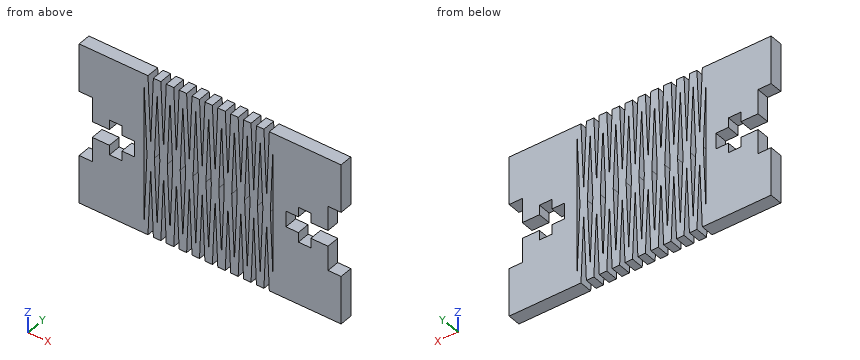
```python
from build123d import *

# Parameters (mm, degrees)
SKETCH1_W            = 61
SKETCH1_H            = 37.5
BOSS_EXTRUDE1_DEPTH  = 3
CUT_EXTRUDE2_DEPTH   = 36.927879147
MIRROR2_COPY_1_DEPTH = 36.927879147
CUT_EXTRUDE3_DEPTH   = 36.927879147
LPATTERN1_COUNT      = 10
LPATTERN1_PITCH      = 3


with BuildPart() as part:
    # Sketch1 → Boss-Extrude1 (new body)
    with BuildSketch(Plane(origin=(0, 0, 0), x_dir=(1, 0, 0), z_dir=(0, 1, 0))):
        Rectangle(SKETCH1_W, SKETCH1_H)
    extrude(amount=BOSS_EXTRUDE1_DEPTH)

    # Sketch3 → Cut-Extrude2 (cut, through all)
    with BuildSketch(Plane(origin=(0, 3, 0), x_dir=(1, 0, 0), z_dir=(0, 1, 0))):
        Polygon((30.5, 7.55), (27.45, 7.55), (27.45, 1.85), (23.45, 1.85), (23.45, 4.1), (20.55, 4.1), (20.55, 1.85), (17.65, 1.85), (17.65, 0), (30.5, 0), align=None)
    cut_extrude2 = extrude(amount=-CUT_EXTRUDE2_DEPTH, mode=Mode.SUBTRACT)

    # Mirror1: Cut-Extrude2 across plane
    add(cut_extrude2.mirror(Plane.XY), mode=Mode.SUBTRACT)

    # Mirror2: Cut-Extrude2 across plane
    add(cut_extrude2.mirror(Plane(origin=(0, 0, 0), x_dir=(0, 0, 1), z_dir=(1, 0, 0))), mode=Mode.SUBTRACT)

    # Mirror2 copy 1 sketch → Mirror2 copy 1 (cut, through all)
    with BuildSketch(Plane(origin=(0, 3, 0), x_dir=(-1, 0, 0), z_dir=(0, 1, 0))):
        Polygon((30.5, 7.55), (27.45, 7.55), (27.45, 1.85), (23.45, 1.85), (23.45, 4.1), (20.55, 4.1), (20.55, 1.85), (17.65, 1.85), (17.65, 0), (30.5, 0), align=None)
    extrude(amount=-MIRROR2_COPY_1_DEPTH, mode=Mode.SUBTRACT)

    # Sketch4 → Cut-Extrude3 (cut, through all)
    with BuildSketch(Plane(origin=(0, 3, 0), x_dir=(1, 0, 0), z_dir=(0, 1, 0))):
        Polygon((14.65, 15.575), (14.65, -15.575), (14.0229932, 0), align=None)
        Polygon((13.7770068, 18.75), (13.15, 3.175), (12.5229932, 18.75), align=None)
        Polygon((13.15, -3.175), (12.5229932, -18.75), (13.7770068, -18.75), align=None)
        Polygon((11.65, 15.575), (11.65, -15.575), (12.2770068, 0), align=None)
    cut_extrude3 = extrude(amount=-CUT_EXTRUDE3_DEPTH, mode=Mode.SUBTRACT)

    # LPattern1: Cut-Extrude3 ×10
    with Locations(*[(-i * LPATTERN1_PITCH, 0, 0) for i in range(1, LPATTERN1_COUNT)]):
        add(cut_extrude3, mode=Mode.SUBTRACT)


solid = part.part
```
Could you check a few things on this model? Use its own coordinates, in mm. Coordinates: 2 decimals unless noted, no trailing zeros. Loops run counter-clockwise (first coordinate to the right, second up) from the corner with the lowest first, then second, coordinate; pieces in that order, holes last. Notation, with made-up numbers: M -37,6 L -28,6 A20 cw -28,35 Z; hole C 66.25,-1 d7. An arc over 180 degrees is marked long. Put each result on its own line as item: value. Start each with the question number.
(1) Suppose I cut it at B-B on y = 1.95. Count the separate pieces of the cut face and the enclosed holes in it, then the cut area to 3 significant figures.
(2) Will this pin go through, and if not, where does the flat tip stop? P1, Ø1.1, axis at y = 1, z = 3, coming from the +X side.
(3) Suppose I cut it at A-A on x = -26. Please give me the cut outline in (y, z), then the cut area to 3 significant figures.
(4) I need wall thicknesses on line 1 (Z direction, x = -23.5, y = 1). Which ranges of the line are inside material? Lowest first, please. Write a range as from..to.
Solutions:
1. separate pieces: 1
1. enclosed holes: 11
1. area: 1,710 mm2
2. P1: stops at x = 27.45
3. outline: M 0,-18.75 L 3,-18.75 L 3,-1.85 L 0,-1.85 Z; M 0,1.85 L 3,1.85 L 3,18.75 L 0,18.75 Z
3. area: 101 mm2
4. line 1: z = -18.75..-1.85, 1.85..18.75
